Design review of the part built by this model. Coordinates are the model's own, in mm. A direction names the side the tool comes from. Round coordinates to 2 decimals unless told otherwise and drop trailing zeros. Order: outer loops, then holes, each group sorted by start corner. A loop starts at its lowest first (then second) coordinate and runs counter-clockwise, first axis right, second up. Notation, with made-up numbers: (46, 48.25) - (105, 48.25) arc R27 cw to (105, 85.25) - close; hole circle Ø11 at (-6.5, 55). An arc over 180 degrees is marked (long way). Answer as a JSON object with one key per item and string values. Group by question number.
from build123d import *

# Parameters (mm, degrees)
F1_DEPTH = 2
F2_R     = 1
F3_DEPTH = 25


with BuildPart() as f1:
    # F0 (on Top) → F1 (new body)
    with BuildSketch(Plane.XY):
        with BuildLine():
            ThreePointArc((4.941112, -0.76512), (4.985256, -0.383692), (5, 0))
            ThreePointArc((5, 0), (4.985256, 0.383692), (4.941112, 0.76512))
            ThreePointArc((4.941112, 0.76512), (4.829629, 1.294095), (4.661689, 1.807943))
            ThreePointArc((4.661689, 1.807943), (4.330127, 2.5), (3.896569, 3.13317))
            ThreePointArc((3.896569, 3.13317), (3.535534, 3.535534), (3.13317, 3.896569))
            ThreePointArc((3.13317, 3.896569), (2.5, 4.330127), (1.807943, 4.661689))
            ThreePointArc((1.807943, 4.661689), (1.294095, 4.829629), (0.76512, 4.941112))
            ThreePointArc((0.76512, 4.941112), (0, 5), (-0.76512, 4.941112))
            ThreePointArc((-0.76512, 4.941112), (-1.294095, 4.829629), (-1.807943, 4.661689))
            ThreePointArc((-1.807943, 4.661689), (-2.5, 4.330127), (-3.13317, 3.896569))
            ThreePointArc((-3.13317, 3.896569), (-3.535534, 3.535534), (-3.896569, 3.13317))
            ThreePointArc((-3.896569, 3.13317), (-4.330127, 2.5), (-4.661689, 1.807943))
            ThreePointArc((-4.661689, 1.807943), (-4.829629, 1.294095), (-4.941112, 0.76512))
            ThreePointArc((-4.941112, 0.76512), (-5, 0), (-4.941112, -0.76512))
            ThreePointArc((-4.941112, -0.76512), (-4.829629, -1.294095), (-4.661689, -1.807943))
            ThreePointArc((-4.661689, -1.807943), (-4.330127, -2.5), (-3.896569, -3.13317))
            ThreePointArc((-3.896569, -3.13317), (-3.535534, -3.535534), (-3.13317, -3.896569))
            ThreePointArc((-3.13317, -3.896569), (-2.5, -4.330127), (-1.807943, -4.661689))
            ThreePointArc((-1.807943, -4.661689), (-1.294095, -4.829629), (-0.76512, -4.941112))
            ThreePointArc((-0.76512, -4.941112), (0, -5), (0.76512, -4.941112))
            ThreePointArc((0.76512, -4.941112), (1.294095, -4.829629), (1.807943, -4.661689))
            ThreePointArc((1.807943, -4.661689), (2.5, -4.330127), (3.13317, -3.896569))
            ThreePointArc((3.13317, -3.896569), (3.535534, -3.535534), (3.896569, -3.13317))
            ThreePointArc((3.896569, -3.13317), (4.330127, -2.5), (4.661689, -1.807943))
            ThreePointArc((4.661689, -1.807943), (4.829629, -1.294095), (4.941112, -0.76512))
        make_face()
        with BuildLine():
            ThreePointArc((4.941112, 0.76512), (4.985256, 0.383692), (5, 0))
            ThreePointArc((5, 0), (4.985256, -0.383692), (4.941112, -0.76512))
            Line((4.941112, -0.76512), (7.841904, 0))
            Line((7.841904, 0), (4.941112, 0.76512))
        make_face()
        with BuildLine():
            ThreePointArc((3.896569, 3.13317), (4.330127, 2.5), (4.661689, 1.807943))
            Line((4.661689, 1.807943), (6.791288, 3.920952))
            Line((6.791288, 3.920952), (3.896569, 3.13317))
        make_face()
        with BuildLine():
            Line((6.791288, -3.920952), (4.661689, -1.807943))
            ThreePointArc((4.661689, -1.807943), (4.330127, -2.5), (3.896569, -3.13317))
            Line((3.896569, -3.13317), (6.791288, -3.920952))
        make_face()
        with BuildLine():
            ThreePointArc((1.807943, 4.661689), (2.5, 4.330127), (3.13317, 3.896569))
            Line((3.13317, 3.896569), (3.920952, 6.791288))
            Line((3.920952, 6.791288), (1.807943, 4.661689))
        make_face()
        with BuildLine():
            Line((3.920952, -6.791288), (3.13317, -3.896569))
            ThreePointArc((3.13317, -3.896569), (2.5, -4.330127), (1.807943, -4.661689))
            Line((1.807943, -4.661689), (3.920952, -6.791288))
        make_face()
        with BuildLine():
            ThreePointArc((-0.76512, 4.941112), (0, 5), (0.76512, 4.941112))
            Line((0.76512, 4.941112), (0, 7.841904))
            Line((0, 7.841904), (-0.76512, 4.941112))
        make_face()
        with BuildLine():
            Line((0, -7.841904), (0.76512, -4.941112))
            ThreePointArc((0.76512, -4.941112), (0, -5), (-0.76512, -4.941112))
            Line((-0.76512, -4.941112), (0, -7.841904))
        make_face()
        with BuildLine():
            ThreePointArc((-3.13317, 3.896569), (-2.5, 4.330127), (-1.807943, 4.661689))
            Line((-1.807943, 4.661689), (-3.920952, 6.791288))
            Line((-3.920952, 6.791288), (-3.13317, 3.896569))
        make_face()
        with BuildLine():
            Line((-3.920952, -6.791288), (-1.807943, -4.661689))
            ThreePointArc((-1.807943, -4.661689), (-2.5, -4.330127), (-3.13317, -3.896569))
            Line((-3.13317, -3.896569), (-3.920952, -6.791288))
        make_face()
        with BuildLine():
            ThreePointArc((-4.661689, 1.807943), (-4.330127, 2.5), (-3.896569, 3.13317))
            Line((-3.896569, 3.13317), (-6.791288, 3.920952))
            Line((-6.791288, 3.920952), (-4.661689, 1.807943))
        make_face()
        with BuildLine():
            Line((-6.791288, -3.920952), (-3.896569, -3.13317))
            ThreePointArc((-3.896569, -3.13317), (-4.330127, -2.5), (-4.661689, -1.807943))
            Line((-4.661689, -1.807943), (-6.791288, -3.920952))
        make_face()
        with BuildLine():
            ThreePointArc((-4.941112, -0.76512), (-5, 0), (-4.941112, 0.76512))
            Line((-4.941112, 0.76512), (-7.841904, 0))
            Line((-7.841904, 0), (-4.941112, -0.76512))
        make_face()
    extrude(amount=F1_DEPTH)

    # F2 (on face) → F3 (cut)
    with BuildSketch(Plane.XY.offset(2)):
        Circle(F2_R)
    extrude(amount=-F3_DEPTH, mode=Mode.SUBTRACT)


solid = f1.part
1. To check wall thickness, follow line 1 (Y direction, x = 5.5, z = 1.15); line 2 (X direction, y = -5, z = 1.05); line 3 (X direction, y = 2.5, z = 0.8). State the ranges of each line that lie inside material, in increasing order. Write a range as from..to.
2. Clearance check with a flat-ended pin moving along its axis: P1, Ø1.2, axis at x = 0, y = 0, coming from the -Z side. State where the tip first meets the part, or that it passes through.
3. Take a section at A-A, the plane x = -0.5. Give the boundary of the cut face in (y, z), then the cut area to 3 significant figures.
4. Tool access review of faces 5 (the flat face through (-5.32, 3.52, 0.99)), 6 (the flat face through (-5.71, -2.85, 0.99)), 7 (the flat face through (6.412, 0.377, 0.986)): name each direction out of +Z, -Z, +X, -X, +Y, -Y from which nothing blocks a thin tool from reaching the whole face with its end or side.
5. Take a section at B-B, the plane x = 2.5. Give the boundary of the cut face in (y, z).
6. Mouldability with a two-part tool opening along Y and no side actions: class faces 1 (the flat face through (-5.36, -3.53, 0.99)), 2 (the flat face through (0.39, 6.37, 0.99)), 3 (the flat face through (-3.52, -5.32, 0.99)), 4 (the flat face through (3.53, -5.36, 0.99)) as pulls with the +Y half, pulls with the -Y half, needs draft (parallel to the pull), parting line crosses it, or undercut.
Response values:
{
 "1": {"line 1": "-3.57..-2.64, -0.62..0.62, 2.64..3.57", "line 2": "-3.43..-2.14, -0.75..0.75, 2.14..3.43", "line 3": "-5.36..5.36"},
 "2": {"P1": "through"},
 "3": {"outline": "(-5.95, 0) - (-0.87, 0) - (-0.87, 2) - (-5.95, 2) - close; (0.87, 0) - (5.95, 0) - (5.95, 2) - (0.87, 2) - close", "area": "20.3 mm2"},
 "4": {"face 5": "+Z, -Z, +Y", "face 6": "+Z, -Z, -X", "face 7": "+Z, -Z, +X"},
 "5": {"outline": "(-5.36, 0) - (5.36, 0) - (5.36, 2) - (-5.36, 2) - close"},
 "6": {"face 1": "pulls with the -Y half", "face 2": "pulls with the +Y half", "face 3": "undercut", "face 4": "undercut"}
}
